Design review of the part shown in the three views and the two pictorial views. Dimensions are in mm from the part's minimum x, y and z. Give positions to 0.01 mm unless a question says otherwise; leave off trailing zeros. Order: outer loops, then holes, each group sorted by start corner. A loop starts at its lowest first (then second) coordinate and runs counter-clockwise, first axis right, second up.
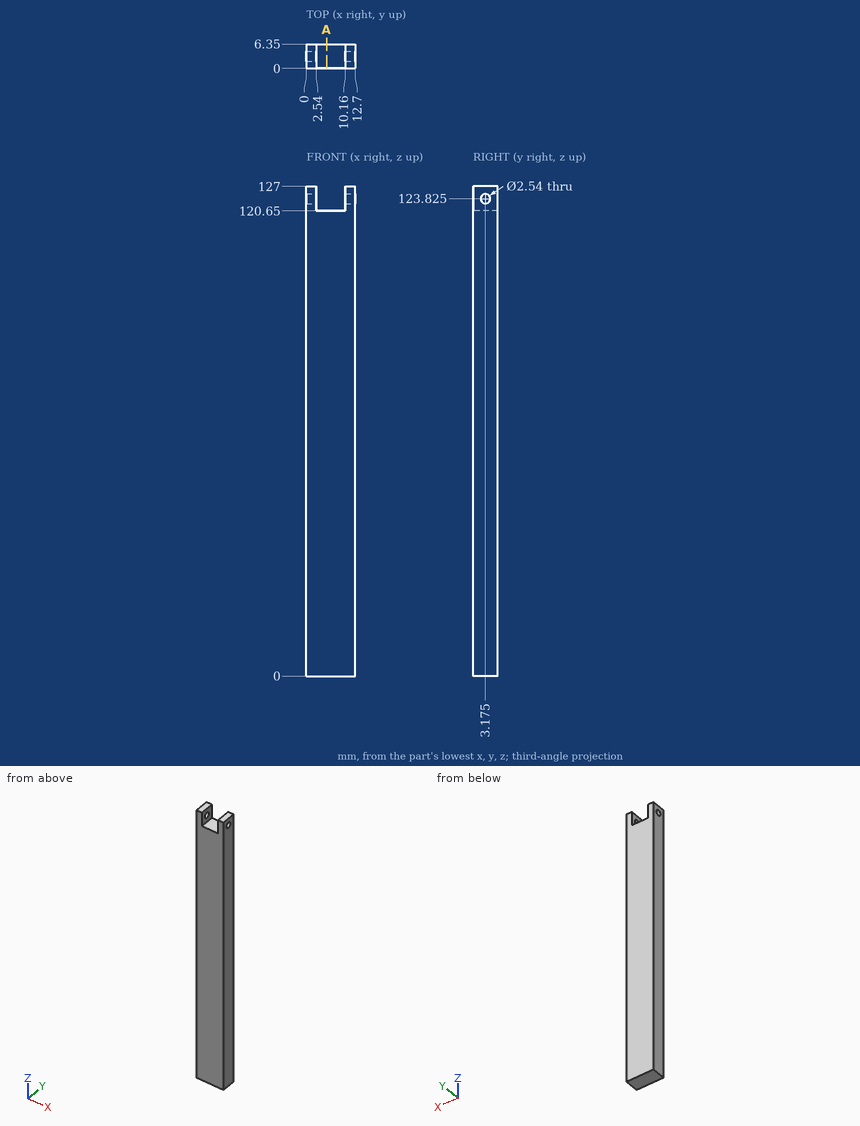
1) To check wall thickness, follow line 1 (X direction, y = 6, z = 121); line 2 (Z direction, x = 8, y = 0.75); line 3 (Z direction, x = 2.5, y = 2.75). State the ranges of each line that lie inside material, in increasing order.
Answer sheet:
line 1: x = 0 to 2.54, 10.16 to 12.7
line 2: z = 0 to 120.65
line 3: z = 0 to 122.63, 125.02 to 127
2) Clearance check with a flat-ended pin moving along its axis: pin 1 (3 mm diameter, centred on x = 7.5, y = 2.5, fed in from +Z). State where the tip first meets the part, or that it passes through.
Answer sheet:
pin 1: stops at z = 120.65
3) We need section A-A on x = 5.25. Give the boundary of the cut face in (y, z), then the cut area to 3 significant figures.
Answer sheet:
outline: (0, 0) - (6.35, 0) - (6.35, 120.65) - (0, 120.65) - close
area: 766 mm2
